The model under review builds one solid part; all positions refer to its coordinate system, in mm. Coordinates: 2 decimals unless noted, no trailing zeros. Write each loop counter-clockwise with the first axis right and the second up, starting at its lowest first coordinate (ties: lowest second). Pieces come first, ordered by that corner, then holes. Notation, with made-up numbers: (33, 44.5) - (82, 44.5) arc R19 ccw to (82, 52.5) - close; hole circle Ø3 at (-21.5, 66.25). An arc over 180 degrees is marked (long way). Put each result on its own line as item: value. Start each with the question number.
Item 1: To check wall thickness, follow L1, parallel to X at y = 2.55, z = -31.79; L2, parallel to X at y = 2.7, z = -24.29; L3, parallel to Z at x = 0, y = 2.25. State the ranges of each line that lie inside material, in increasing order. Write a range as [from, to].
Item 2: Consider section A-A on y = 2.8. State how many separate pieces and enclosed holes the cut face has, then the cut area to 3 significant figures.
Item 3: Consider section B-B on x = 25.5. Give the boundary of the cut face in (y, z).
Item 4: For pin 1 (2.5 mm diameter, centred on x = -7.57, z = 20.54, fed in from -Y); pin 2 (1 mm diameter, centred on x = -23, y = 3, fed in from -Z), all flat-tipped, find the tip position at first contact; note any pin that passes through.
Item 5: Consider section C-C on x = -27. Give the boundary of the cut face in (y, z).
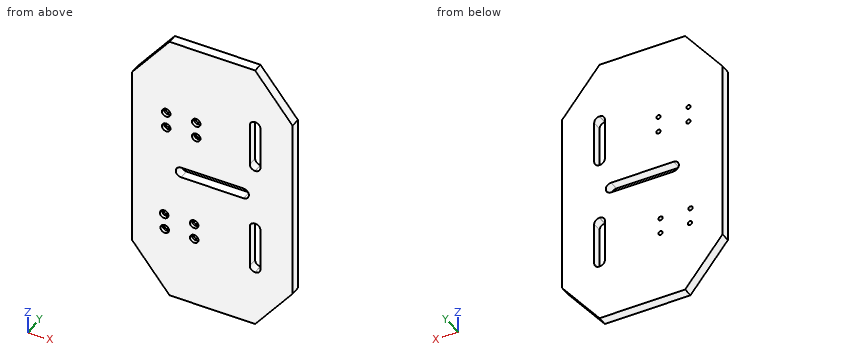
```python
from build123d import *

# Parameters (mm, degrees)
BOSS_EXTRUDE1_DEPTH = 4.5
CUT_EXTRUDE2_DEPTH  = 10
SKETCH7_R           = 1
CUT_EXTRUDE3_DEPTH  = 5
SKETCH11_R          = 2
SKETCH11_R_2        = 1
CUT_EXTRUDE4_DEPTH  = 1.65


with BuildPart() as part:
    # Sketch1 → Boss-Extrude1 (new body)
    with BuildSketch(Plane(origin=(0, 0, 0), x_dir=(1, 0, 0), z_dir=(0, 1, 0))):
        Polygon((-37.5, -43.117707706), (-20.011895516, -65), (20.011895516, -65), (37.5, -43.117707706), (37.5, 43.117707706), (20.011895516, 65), (-20.011895516, 65), (-37.5, 43.117707706), align=None)
    extrude(amount=BOSS_EXTRUDE1_DEPTH)

    # Sketch5 → Cut-Extrude2 (cut)
    with BuildSketch(Plane(origin=(0, 4.5, 0), x_dir=(1, 0, 0), z_dir=(0, 1, 0))):
        with BuildLine():
            Line((-14.620176413, -2.5), (14.620176413, -2.5))
            ThreePointArc((14.620176413, -2.5), (16.352588027, -1.782411614), (17.070176413, -0.05))
            Line((17.070176413, -0.05), (17.070176413, 0.05))
            ThreePointArc((17.070176413, 0.05), (16.352588027, 1.782411614), (14.620176413, 2.5))
            Line((14.620176413, 2.5), (-14.620176413, 2.5))
            ThreePointArc((-14.620176413, 2.5), (-16.352588027, 1.782411614), (-17.070176413, 0.05))
            Line((-17.070176413, 0.05), (-17.070176413, -0.05))
            ThreePointArc((-17.070176413, -0.05), (-16.352588027, -1.782411614), (-14.620176413, -2.5))
        make_face()
        with BuildLine():
            Line((19.95, -38.5), (20.05, -38.5))
            ThreePointArc((20.05, -38.5), (21.782411614, -37.782411614), (22.5, -36.05))
            Line((22.5, -36.05), (22.5, -15.95))
            ThreePointArc((22.5, -15.95), (21.782411614, -14.217588386), (20.05, -13.5))
            Line((20.05, -13.5), (19.95, -13.5))
            ThreePointArc((19.95, -13.5), (18.217588386, -14.217588386), (17.5, -15.95))
            Line((17.5, -15.95), (17.5, -36.05))
            ThreePointArc((17.5, -36.05), (18.217588386, -37.782411614), (19.95, -38.5))
        make_face()
        with BuildLine():
            Line((19.95, 13.5), (20.05, 13.5))
            ThreePointArc((20.05, 13.5), (21.782411614, 14.217588386), (22.5, 15.95))
            Line((22.5, 15.95), (22.5, 36.05))
            ThreePointArc((22.5, 36.05), (21.782411614, 37.782411614), (20.05, 38.5))
            Line((20.05, 38.5), (19.95, 38.5))
            ThreePointArc((19.95, 38.5), (18.217588386, 37.782411614), (17.5, 36.05))
            Line((17.5, 36.05), (17.5, 15.95))
            ThreePointArc((17.5, 15.95), (18.217588386, 14.217588386), (19.95, 13.5))
        make_face()
    extrude(amount=-CUT_EXTRUDE2_DEPTH, mode=Mode.SUBTRACT)

    # Sketch7 → Cut-Extrude3 (cut)
    with BuildSketch(Plane(origin=(0, 4.5, 0), x_dir=(1, 0, 0), z_dir=(0, 1, 0))):
        with Locations((-8.5, 24.29)):
            Circle(SKETCH7_R)
        with Locations((-22.5, 24.29)):
            Circle(SKETCH7_R)
        with Locations((-22.26760758, 31.79)):
            Circle(SKETCH7_R)
        with Locations((-21.57, -20.54)):
            Circle(SKETCH7_R)
        with Locations((-21.57, -28.04)):
            Circle(SKETCH7_R)
        with Locations((-7.57, -28.04)):
            Circle(SKETCH7_R)
        with Locations((-7.57, -20.54)):
            Circle(SKETCH7_R)
        with Locations((-8.5, 31.79)):
            Circle(SKETCH7_R)
    extrude(amount=-CUT_EXTRUDE3_DEPTH, mode=Mode.SUBTRACT)

    # Sketch11 → Cut-Extrude4 (cut)
    with BuildSketch(Plane.XZ):
        with Locations((-7.57, 20.54)):
            Circle(SKETCH11_R)
        with Locations((-7.57, 20.54)):
            Circle(SKETCH11_R_2, mode=Mode.SUBTRACT)
        with Locations((-21.57, 20.54)):
            Circle(SKETCH11_R)
        with Locations((-21.57, 20.54)):
            Circle(SKETCH11_R_2, mode=Mode.SUBTRACT)
        with Locations((-8.5, -24.29)):
            Circle(SKETCH11_R)
        with Locations((-8.5, -24.29)):
            Circle(SKETCH11_R_2, mode=Mode.SUBTRACT)
        with Locations((-8.5, -31.79)):
            Circle(SKETCH11_R)
        with Locations((-8.5, -31.79)):
            Circle(SKETCH11_R_2, mode=Mode.SUBTRACT)
        with Locations((-7.57, 28.04)):
            Circle(SKETCH11_R)
        with Locations((-21.57, 28.04)):
            Circle(SKETCH11_R)
        with Locations((-22.26760758, -31.79)):
            Circle(SKETCH11_R)
        with Locations((-22.5, -24.29)):
            Circle(SKETCH11_R)
    extrude(amount=-CUT_EXTRUDE4_DEPTH, mode=Mode.SUBTRACT)


solid = part.part
```
Report:
1. L1: [-37.5, -23.27], [-21.27, -9.5], [-7.5, 17.5], [22.5, 37.5]
1. L2: [-37.5, -23.5], [-21.5, -9.5], [-7.5, 17.5], [22.5, 37.5]
1. L3: [-65, -2.5], [2.5, 65]
2. separate pieces: 1
2. enclosed holes: 11
2. area: 8,550 mm²
3. outline: (0, -58.13) - (4.5, -58.13) - (4.5, 58.13) - (0, 58.13) - close
4. pin 1: y = 1.65
4. pin 2: z = -61.89
5. outline: (0, -56.26) - (4.5, -56.26) - (4.5, 56.26) - (0, 56.26) - close
